Geometry check sheet. Reference: the model listing, model coordinates, mm. Round coordinates to 2 decimals unless told otherwise and drop trailing zeros. Order: outer loops, then holes, each group sorted by start corner. A loop starts at its lowest first (then second) coordinate and runs counter-clockwise, first axis right, second up. Notation, with made-up numbers: (85, 62) - (125, 62) arc R15 cw to (125, 75) - close; hole circle Ø3 at (-40, 13). An arc over 180 degrees is marked (long way). Use a Markdown table: item, result. Add a question column.
(1) Section check B-B on z = 3.65. Record the boundary of the cut face in (x, y).
(2) Thickness scan on line 1 along X through (y, z) = (0.1, 1.5); line 2 along Y through (x, z) = (6, 2.65); line 3 along X through (y, z) = (-1.3, 0.5). Record the ranges inside material, lowest first. Write a range as [from, to].
(3) Mould release check, pull along X, two halves, no side actions. Record for faces 1 (the face through (-10, -2.5, 2)), 2 (the face through (-26.18, -1.08, 2.46)), 3 (the face through (8.5, 0.1, 2.5)), 4 (the face through (7.48, 0.61, 2.46)): released by +X, released by -X, zero draft, split by the parting line, or undercut.
(4) Section check A-A on y = 0. Record the boundary of the cut face in (x, z).
(5) Section check C-C on y = -1.3. Record the boundary of the cut face in (x, z).
(6) Gauge pin test, flat end, axial feed: P1, Ø3, axis at x = -25, y = 0, coming from the +Z side. Record the tip position at first contact, or that the pin passes through.
Autodesk Fusion 360 part; units mm, degrees
sketch "스케치1" plane through (0, 0, 0) normal (0, 0, 1) x (1, 0, 0)
  line L0 (-25, -2.5) -> (6, -2.5)
  arc A0 (6, -2.5) -> (6, 2.5) centre (6, 0) ccw
  line L1 (6, 2.5) -> (-25, 2.5)
  arc A1 (-25, 2.5) -> (-25, -2.5) centre (-25, 0) ccw
  line L2 (-25, 0) -> (6, 0) construction
  circle A2 centre (6, 0) radius 1.6
  circle A3 centre (-25, 0) radius 1.6
  dimension "d1" = 31
  dimension "d2" = 5
  dimension "d3" = 3.2
  dimension "d4" = 3.2
extrude "돌출1" add sketch "스케치1" along normal blind 5
Check sheet entries:
| question | item | result |
|---|---|---|
| 1 | outline | (-25, -2.5) - (6, -2.5) arc R2.5 ccw to (6, 2.5) - (-25, 2.5) arc R2.5 ccw to start; hole circle Ø3.2 at (-25, 0); hole circle Ø3.2 at (6, 0) |
| 2 | line 1 | x = [-27.5, -26.6], [-23.4, 4.4], [7.6, 8.5] |
| 2 | line 2 | y = [-2.5, -1.6], [1.6, 2.5] |
| 2 | line 3 | x = [-27.14, -25.93], [-24.07, 5.07], [6.93, 8.14] |
| 3 | face 1 | zero draft |
| 3 | face 2 | undercut |
| 3 | face 3 | released by +X |
| 3 | face 4 | undercut |
| 4 | outline | (-27.5, 0) - (-26.6, 0) - (-26.6, 5) - (-27.5, 5) - close; (-23.4, 0) - (4.4, 0) - (4.4, 5) - (-23.4, 5) - close; (7.6, 0) - (8.5, 0) - (8.5, 5) - (7.6, 5) - close |
| 5 | outline | (-27.14, 0) - (-25.93, 0) - (-25.93, 5) - (-27.14, 5) - close; (-24.07, 0) - (5.07, 0) - (5.07, 5) - (-24.07, 5) - close; (6.93, 0) - (8.14, 0) - (8.14, 5) - (6.93, 5) - close |
| 6 | P1 | passes through |
